Work out the finished part from the listing and answer in its coordinate system (mm). Face numbers are marked on the shaded views. A direction names the side the tool comes from. Round coordinates to 2 decimals unless told otherwise and drop trailing zeros. Loops run counter-clockwise (first coordinate to the right, second up) from the corner with the lowest first, then second, coordinate; pieces in that order, holes last. Notation, with made-up numbers: (89, -20) - (126, -20) arc R4 cw to (126, -14) - close; hole circle Ø11 at (-32.75, -36). An arc over 180 degrees is marked (long way). Answer as CSV lines item,"result". Start each with the question number.
Q1. Section C-C on y = 14.5 is taken. Write down the section's boundary in (x, z).
Q2. The mould has two halves that part along X. Classify the marked faces 1, 2 and 3: +X half, -X half, draft (parallel to the pull), parting line (faces both ways), or undercut.
Q3. Section A-A on x = 52.5 is taken. Write down the section's boundary in (y, z).
Q4. For the marked faces 4 and 5, determine the directions among +Z, -Z, +X, -X, +Y, -Y from which every point of the face is accessible in a straight line to the end or side of a thin tool.
Q5. Each of these flat-tipped pins is pushed along its axis until it touches: pin 1 Ø1 at (y, z) = (13.5, -9.5) entering from -X; pin 2 Ø9 at (y, z) = (16.5, -0.5) entering from +X; pin 3 Ø2 at (x, z) = (-41, -15) entering from -Y. Where does it stop, or does it pass through?
Q6. Section D-D on x = -14 is taken. Write down the section's boundary in (y, z).
Q7. Straight lines are drawn through the part: L1, parallel to Z at x = 52.5, y = 3; L2, parallel to X at y = 5.25, z = 42.5; L3, parallel to Z at x = -40, y = 8.75. For each, find the intervals that lie inside material, in ascending order. Write a range as [from, to].
Q8. Section B-B on z = 42.5 is taken. Write down the section's boundary in (x, y).
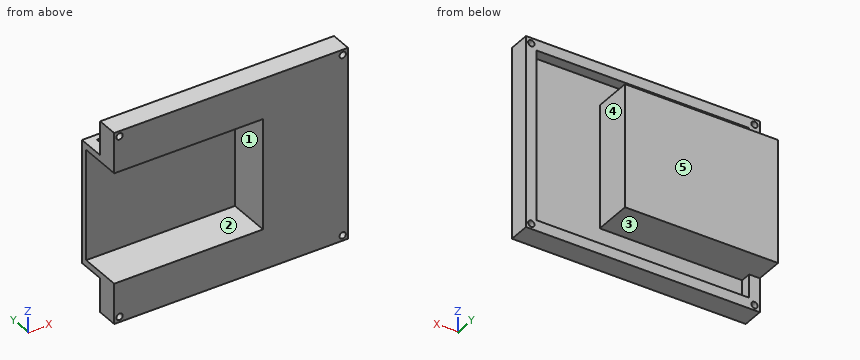
```python
from build123d import *

# Parameters (mm, degrees)
SKETCH1_W            = 110
SKETCH1_H            = 90
BOSS_EXTRUDE2_DEPTH  = 5
SKETCH2_W            = 110
SKETCH2_H            = 5
BOSS_EXTRUDE4_DEPTH  = 25
SKETCH3_W            = 110
SKETCH3_H            = 5
BOSS_EXTRUDE5_DEPTH  = 25
SKETCH5_W            = 5
SKETCH5_H            = 80
BOSS_EXTRUDE6_DEPTH  = 25
SKETCH8_W            = 72
SKETCH8_H            = 58
BOSS_EXTRUDE7_DEPTH  = 25
SKETCH10_W           = 52
SKETCH10_H           = 20.115523146
CUT_EXTRUDE1_DEPTH   = 70
SKETCH11_W           = 90
SKETCH11_H           = 7
CUT_EXTRUDE2_DEPTH   = 110
SKETCH12_R           = 1.5
CUT_EXTRUDE3_DEPTH   = 23
SKETCH13_R           = 1.5
CUT_EXTRUDE4_DEPTH   = 23
SKETCH14_R           = 1.5
CUT_EXTRUDE5_DEPTH   = 23
SKETCH15_R           = 1.5
CUT_EXTRUDE6_DEPTH   = 23
SKETCH18_W           = 5
SKETCH18_H           = 13
CUT_EXTRUDE7_DEPTH   = 110
SKETCH19_W           = 5
SKETCH19_H           = 13
CUT_EXTRUDE13_DEPTH  = 85
SKETCH26_W           = 5
SKETCH26_H           = 13
CUT_EXTRUDE17_DEPTH  = 105
SKETCH29_W           = 5
SKETCH29_H           = 11
BOSS_EXTRUDE14_DEPTH = 5
SKETCH30_W           = 5
SKETCH30_H           = 11
BOSS_EXTRUDE15_DEPTH = 5
SKETCH34_W           = 2.5
SKETCH34_H           = 2.5
CUT_EXTRUDE18_DEPTH  = 3
SKETCH37_W           = 72
SKETCH37_H           = 13
CUT_EXTRUDE20_DEPTH  = 58
SKETCH39_W           = 72
SKETCH39_H           = 3
BOSS_EXTRUDE17_DEPTH = 13
SKETCH41_W           = 2
SKETCH41_H           = 55
BOSS_EXTRUDE18_DEPTH = 13
SKETCH43_W           = 70
SKETCH43_H           = 3
BOSS_EXTRUDE19_DEPTH = 13
SKETCH44_W           = 70
SKETCH44_H           = 52
BOSS_EXTRUDE22_DEPTH = 3
SKETCH55_W           = 2.5
SKETCH55_H           = 2.5
CUT_EXTRUDE25_DEPTH  = 3


with BuildPart() as part:
    # Sketch1 → Boss-Extrude2 (new body)
    with BuildSketch(Plane(origin=(0, 0, 0), x_dir=(1, 0, 0), z_dir=(0, 1, 0))):
        Rectangle(SKETCH1_W, SKETCH1_H)
    extrude(amount=BOSS_EXTRUDE2_DEPTH)

    # Sketch2 → Boss-Extrude4 (add)
    with BuildSketch(Plane(origin=(0, 5, 0), x_dir=(1, 0, 0), z_dir=(0, 1, 0))):
        with Locations((0, 42.5)):
            Rectangle(SKETCH2_W, SKETCH2_H)
    extrude(amount=BOSS_EXTRUDE4_DEPTH)

    # Sketch3 → Boss-Extrude5 (add)
    with BuildSketch(Plane(origin=(0, 5, 0), x_dir=(1, 0, 0), z_dir=(0, 1, 0))):
        with Locations((0, -42.5)):
            Rectangle(SKETCH3_W, SKETCH3_H)
    extrude(amount=BOSS_EXTRUDE5_DEPTH)

    # Sketch5 → Boss-Extrude6 (add)
    with BuildSketch(Plane(origin=(0, 5, 0), x_dir=(1, 0, 0), z_dir=(0, 1, 0))):
        with Locations((52.5, 0)):
            Rectangle(SKETCH5_W, SKETCH5_H)
    extrude(amount=BOSS_EXTRUDE6_DEPTH)

    # Sketch8 → Boss-Extrude7 (add)
    with BuildSketch(Plane(origin=(0, 5, 0), x_dir=(1, 0, 0), z_dir=(0, 1, 0))):
        with Locations((-19, 0)):
            Rectangle(SKETCH8_W, SKETCH8_H)
    extrude(amount=BOSS_EXTRUDE7_DEPTH)

    # Sketch10 → Cut-Extrude1 (cut)
    with BuildSketch(Plane.ZY.offset(55)):
        with Locations((0, 10.057761573)):
            Rectangle(SKETCH10_W, SKETCH10_H)
    extrude(amount=-CUT_EXTRUDE1_DEPTH, mode=Mode.SUBTRACT)

    # Sketch11 → Cut-Extrude2 (cut)
    with BuildSketch(Plane.ZY.offset(55)):
        with Locations((0, 26.5)):
            Rectangle(SKETCH11_W, SKETCH11_H)
    extrude(amount=-CUT_EXTRUDE2_DEPTH, mode=Mode.SUBTRACT)

    # Sketch12 → Cut-Extrude3 (cut)
    with BuildSketch(Plane(origin=(0, 23, 0), x_dir=(1, 0, 0), z_dir=(0, 1, 0))):
        with Locations((52.5, -42.5)):
            Circle(SKETCH12_R)
    extrude(amount=-CUT_EXTRUDE3_DEPTH, mode=Mode.SUBTRACT)

    # Sketch13 → Cut-Extrude4 (cut)
    with BuildSketch(Plane(origin=(0, 23, 0), x_dir=(1, 0, 0), z_dir=(0, 1, 0))):
        with Locations((-52.5, -42.5)):
            Circle(SKETCH13_R)
    extrude(amount=-CUT_EXTRUDE4_DEPTH, mode=Mode.SUBTRACT)

    # Sketch14 → Cut-Extrude5 (cut)
    with BuildSketch(Plane(origin=(0, 23, 0), x_dir=(1, 0, 0), z_dir=(0, 1, 0))):
        with Locations((52.5, 42.5)):
            Circle(SKETCH14_R)
    extrude(amount=-CUT_EXTRUDE5_DEPTH, mode=Mode.SUBTRACT)

    # Sketch15 → Cut-Extrude6 (cut)
    with BuildSketch(Plane(origin=(0, 23, 0), x_dir=(1, 0, 0), z_dir=(0, 1, 0))):
        with Locations((-52.5, 42.5)):
            Circle(SKETCH15_R)
    extrude(amount=-CUT_EXTRUDE6_DEPTH, mode=Mode.SUBTRACT)

    # Sketch18 → Cut-Extrude7 (cut)
    with BuildSketch(Plane.ZY.offset(55)):
        with Locations((-42.5, 16.5)):
            Rectangle(SKETCH18_W, SKETCH18_H)
    extrude(amount=-CUT_EXTRUDE7_DEPTH, mode=Mode.SUBTRACT)

    # Sketch19 → Cut-Extrude13 (cut)
    with BuildSketch(Plane(origin=(0, 0, -40), x_dir=(-1, 0, 0), z_dir=(0, 0, -1))):
        with Locations((-52.5, 16.5)):
            Rectangle(SKETCH19_W, SKETCH19_H)
    extrude(amount=-CUT_EXTRUDE13_DEPTH, mode=Mode.SUBTRACT)

    # Sketch26 → Cut-Extrude17 (cut)
    with BuildSketch(Plane(origin=(50, 0, 0), x_dir=(0, 0, -1), z_dir=(1, 0, 0))):
        with Locations((-42.5, 16.5)):
            Rectangle(SKETCH26_W, SKETCH26_H)
    extrude(amount=-CUT_EXTRUDE17_DEPTH, mode=Mode.SUBTRACT)

    # Sketch29 → Boss-Extrude14 (add)
    with BuildSketch(Plane(origin=(0, 5, 0), x_dir=(1, 0, 0), z_dir=(0, 1, 0))):
        with Locations((-52.5, 34.5)):
            Rectangle(SKETCH29_W, SKETCH29_H)
    extrude(amount=BOSS_EXTRUDE14_DEPTH)

    # Sketch30 → Boss-Extrude15 (add)
    with BuildSketch(Plane(origin=(0, 5, 0), x_dir=(1, 0, 0), z_dir=(0, 1, 0))):
        with Locations((-52.5, -34.5)):
            Rectangle(SKETCH30_W, SKETCH30_H)
    extrude(amount=BOSS_EXTRUDE15_DEPTH)

    # Sketch34 → Cut-Extrude18 (cut)
    with BuildSketch(Plane.XY.offset(29)):
        with Locations((-48.75, 18.75)):
            Rectangle(SKETCH34_W, SKETCH34_H)
    extrude(amount=-CUT_EXTRUDE18_DEPTH, mode=Mode.SUBTRACT)

    # Sketch37 → Cut-Extrude20 (cut)
    with BuildSketch(Plane.XY.offset(29)):
        with Locations((-19, 16.5)):
            Rectangle(SKETCH37_W, SKETCH37_H)
    extrude(amount=-CUT_EXTRUDE20_DEPTH, mode=Mode.SUBTRACT)

    # Sketch39 → Boss-Extrude17 (add)
    with BuildSketch(Plane(origin=(0, 10, 0), x_dir=(1, 0, 0), z_dir=(0, 1, 0))):
        with Locations((-19, 27.5)):
            Rectangle(SKETCH39_W, SKETCH39_H)
    extrude(amount=BOSS_EXTRUDE17_DEPTH)

    # Sketch41 → Boss-Extrude18 (add)
    with BuildSketch(Plane(origin=(0, 10, 0), x_dir=(1, 0, 0), z_dir=(0, 1, 0))):
        with Locations((16, -1.5)):
            Rectangle(SKETCH41_W, SKETCH41_H)
    extrude(amount=BOSS_EXTRUDE18_DEPTH)

    # Sketch43 → Boss-Extrude19 (add)
    with BuildSketch(Plane(origin=(0, 10, 0), x_dir=(1, 0, 0), z_dir=(0, 1, 0))):
        with Locations((-20, -27.5)):
            Rectangle(SKETCH43_W, SKETCH43_H)
    extrude(amount=BOSS_EXTRUDE19_DEPTH)

    # Sketch44 → Boss-Extrude22 (add)
    with BuildSketch(Plane(origin=(0, 23, 0), x_dir=(1, 0, 0), z_dir=(0, 1, 0))):
        with Locations((-20, 0)):
            Rectangle(SKETCH44_W, SKETCH44_H)
    extrude(amount=-BOSS_EXTRUDE22_DEPTH)

    # Sketch55 → Cut-Extrude25 (cut)
    with BuildSketch(Plane.XY.offset(29)):
        with Locations((-48.75, 18.75)):
            Rectangle(SKETCH55_W, SKETCH55_H)
    extrude(amount=-CUT_EXTRUDE25_DEPTH, mode=Mode.SUBTRACT)


solid = part.part
```
Findings:
1,outline,"(-55, -29) - (17, -29) - (17, 29) - (-55, 29) - (-55, 26) - (15, 26) - (15, -26) - (-55, -26) - close"
2,face 1,"-X half"
2,face 2,"draft"
2,face 3,"undercut"
3,outline,"(0, -45) - (10, -45) - (10, -44) - (0, -44) - close; (0, -41) - (10, -41) - (10, 41) - (0, 41) - close; (0, 44) - (10, 44) - (10, 45) - (0, 45) - close"
4,face 4,"+Y"
4,face 5,"+Z, -Z, +X, -X, +Y"
5,pin 1,"stops at x = 15"
5,pin 2,"stops at x = 17"
5,pin 3,"stops at y = 20"
6,outline,"(0, -45) - (10, -45) - (10, -40) - (5, -40) - (5, -29) - (23, -29) - (23, 29) - (5, 29) - (5, 40) - (10, 40) - (10, 45) - (0, 45) - (0, 26) - (20, 26) - (20, -26) - (0, -26) - close"
7,L1,"z = [-45, -44], [-41, 41], [44, 45]"
7,L2,"x = [-55, -54], [-51, 51], [54, 55]"
7,L3,"z = [-45, -40], [-29, -26], [26, 29], [40, 45]"
8,outline,"(-55, 0) - (-54, 0) - (-54, 10) - (-55, 10) - close; (-51, 0) - (51, 0) - (51, 10) - (-51, 10) - close; (54, 0) - (55, 0) - (55, 10) - (54, 10) - close"
